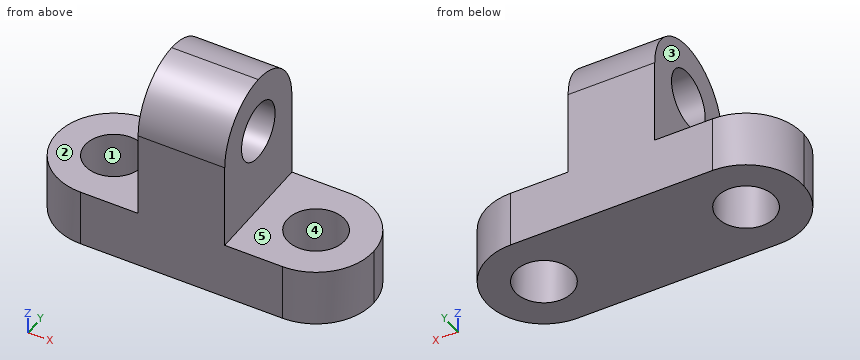
from build123d import *

# Parameters (mm, degrees)
F0_W      = 69.85
F0_H      = 44.45
F1_DEPTH  = 25.4
F2_W      = 25.4
F2_H      = 31.75
F3_DEPTH  = 25.4
F5_DEPTH  = 25.4
F6_R      = 6.35
F7_DEPTH  = 25.4
F9_DEPTH  = 25.4
F11_DEPTH = 25.4
F12_R     = 6.35
F13_DEPTH = 25.4


with BuildPart() as f1:
    # F0 (on Front) → F1 (new body)
    with BuildSketch(Plane.XZ):
        with Locations((34.925, 22.225)):
            Rectangle(F0_W, F0_H)
    extrude(amount=F1_DEPTH)

    # F2 (on face) → F3 (cut)
    with BuildSketch(Plane.XZ.offset(25.4)):
        with Locations((12.7, 28.575)):
            Rectangle(F2_W, F2_H)
        with Locations((57.15, 28.575)):
            Rectangle(F2_W, F2_H)
    extrude(amount=-F3_DEPTH, mode=Mode.SUBTRACT)

    # F4 (on face) → F5 (cut)
    with BuildSketch(Plane.YZ.offset(44.45)):
        with BuildLine():
            ThreePointArc((-25.4, 31.750001), (-21.680256, 40.730257), (-12.7, 44.45))
            Line((-12.7, 44.45), (-25.4, 44.45))
            Line((-25.4, 44.45), (-25.4, 31.750001))
        make_face()
        with BuildLine():
            ThreePointArc((-12.7, 44.45), (-3.719744, 40.730256), (0, 31.75))
            Line((0, 31.75), (0, 44.45))
            Line((0, 44.45), (-12.7, 44.45))
        make_face()
    extrude(amount=-F5_DEPTH, mode=Mode.SUBTRACT)

    # F6 (on face) → F7 (cut)
    with BuildSketch(Plane.YZ.offset(44.45)):
        with Locations((-12.7, 31.75)):
            Circle(F6_R)
    extrude(amount=-F7_DEPTH, mode=Mode.SUBTRACT)

    # F8 (on face) → F9 (cut)
    with BuildSketch(Plane.XY.offset(12.7)):
        with BuildLine():
            ThreePointArc((57.15, 0), (66.130256, -3.719744), (69.85, -12.7))
            Line((69.85, -12.7), (69.85, 0))
            Line((69.85, 0), (57.15, 0))
        make_face()
        with BuildLine():
            ThreePointArc((69.85, -12.7), (66.130256, -21.680256), (57.15, -25.4))
            Line((57.15, -25.4), (69.85, -25.4))
            Line((69.85, -25.4), (69.85, -12.7))
        make_face()
    extrude(amount=-F9_DEPTH, mode=Mode.SUBTRACT)

    # F10 (on face) → F11 (cut)
    with BuildSketch(Plane.XY.offset(12.7)):
        with BuildLine():
            ThreePointArc((0, -12.7), (3.719744, -3.719744), (12.7, 0))
            Line((12.7, 0), (0, 0))
            Line((0, 0), (0, -12.7))
        make_face()
        with BuildLine():
            ThreePointArc((12.7, -25.4), (3.719744, -21.680256), (0, -12.7))
            Line((0, -12.7), (0, -25.4))
            Line((0, -25.4), (12.7, -25.4))
        make_face()
    extrude(amount=-F11_DEPTH, mode=Mode.SUBTRACT)

    # F12 (on face) → F13 (cut)
    with BuildSketch(Plane.XY.offset(12.7)):
        with Locations((12.7, -12.7)):
            Circle(F12_R)
        with Locations((57.15, -12.7)):
            Circle(F12_R)
    extrude(amount=-F13_DEPTH, mode=Mode.SUBTRACT)


solid = f1.part
Source: CAD feature listing. Evaluate the final solid. Frame: model axes, mm. Face numbers are marked on the shaded views. A direction names the side the tool comes from. Round coordinates to 2 decimals unless told otherwise and drop trailing zeros. Write each loop counter-clockwise with the first axis right and the second up, starting at its lowest first coordinate (ties: lowest second). Pieces come first, ordered by that corner, then holes. Notation, with made-up numbers: (89, 13.5) - (136, 13.5) arc R22 cw to (136, 50.5) - close; hole circle Ø3 at (-11, 29). An arc over 180 degrees is marked (long way). Use CSV: the item, a comma, the result in double quotes. Start each with the question number.
(1) Material intervals for probe 1 along Y at (x, z) = (12.7, 8.5); probe 2 along Z at (x, y) = (32.5, -12.7); probe 3 along Z at (x, y) = (49.5, -14.75), sorted ascending. Write a range as [from, to].
(2) Set-up query: the marked faces 4 and 5. Return all of +Z, -Z, +X, -X, +Y, -Y with unobstructed straight access to the full face (end or side cutting, diameter ignored); none if empty.
(3) Cut plane A-A, the plane y = -9.75. Return loops of the section in (x, z), and give its area (3 significant figures).
(4) Cut plane C-C, the plane x = 16. Return loops of the section in (y, z), and give its area (3 significant figures).
(5) Mould query, pull axis X, two halves, no side actions, for the marked faces 1, 2 and 3. Classes: pulls with the +X half, pulls with the -X half, needs draft (parallel to the pull), parting line crosses it, or undercut.
(6) Cut plane B-B, the plane z = 30. Return loops of the section in (x, y), and give its area (3 significant figures).
(7) First-contact query: pin 1 Ø4 at (x, y) = (61.5, -15.5) entering from +Z; pin 2 Ø4 at (y, z) = (-5, 35) entering from +X; pin 3 Ø14.5 at (x, y) = (57.15, -12.7) entering from -Z; pin 4 Ø6 at (x, y) = (46, -3) entering from +Z. Flat tips, straight axial feed; report the tip coordinate or a pass-through.
(8) Cut plane D-D, the plane x = 48. Return loops of the section in (y, z), and give its area (3 significant figures).
Geometry says:
1,probe 1,"[-25.4, -19.05], [-6.35, 0]"
1,probe 2,"[0, 25.4], [38.1, 44.45]"
1,probe 3,"[0, 12.7]"
2,face 4,"+Z, -Z"
2,face 5,"+Z, +X, +Y, -Y"
3,outline,"(0.35, 0) - (7.08, 0) - (7.08, 12.7) - (0.35, 12.7) - close; (18.32, 0) - (51.53, 0) - (51.53, 12.7) - (44.45, 12.7) - (44.45, 26.13) - (25.4, 26.13) - (25.4, 12.7) - (18.32, 12.7) - close; (25.4, 37.37) - (44.45, 37.37) - (44.45, 44.1) - (25.4, 44.1) - close; (62.77, 0) - (69.5, 0) - (69.5, 12.7) - (62.77, 12.7) - close"
3,area,"977 mm²"
4,outline,"(-25.4, 0) - (-18.13, 0) - (-18.13, 12.7) - (-25.4, 12.7) - close; (-7.27, 0) - (0, 0) - (0, 12.7) - (-7.27, 12.7) - close"
4,area,"185 mm²"
5,face 1,"undercut"
5,face 2,"needs draft"
5,face 3,"pulls with the -X half"
6,outline,"(25.4, -25.4) - (44.45, -25.4) - (44.45, -18.8) - (25.4, -18.8) - close; (25.4, -6.6) - (44.45, -6.6) - (44.45, 0) - (25.4, 0) - close"
6,area,"251 mm²"
7,pin 1,"z = 12.7"
7,pin 2,"x = 44.45"
7,pin 3,"z = 0"
7,pin 4,"z = 42.26"
8,outline,"(-25.4, 0) - (0, 0) - (0, 12.7) - (-25.4, 12.7) - close"
8,area,"323 mm²"
